Here's how the part is built. I have some questions about the finished solid (model axes, mm). A direction names the side the tool comes from. Give positions to 0.01 mm unless a question says otherwise; leave off trailing zeros. Write each loop counter-clockwise with the first axis right and the second up, starting at its lowest first coordinate (ties: lowest second). Pieces come first, ordered by that corner, then holes. Notation, with made-up numbers: (-21, 37.5) - (29, 37.5) arc R14 ccw to (29, 64.5) - close; hole circle Ø3 at (87.25, 23.5). An arc over 180 degrees is marked (long way). One line per item, written item: value. Start each with the question number.
1) On a 3-axis mill with a long thin cutter (end or side, diameter ignored), from which of +Z, -Z, +X, -X, +Y, -Y can I reach the whole of each face in a straight line? I mean faces 1 (the flat face through (-45.334, -78, -5)), 2 (the flat face through (-29, -84.507, 1)), 3 (the flat face through (-20, -78, 0.6)), 4 (the flat face through (-47.834, -78, -5)). Say none if no direction works.
2) Please list where these lines run through material, in increasing order: L1, parallel to X at y = -79.5, z = -0.5; L2, parallel to X at y = -72.5, z = 2.25; L3, parallel to Z at x = -19.5, y = -72.5. Write a range as [from, to].
3) I'm going to push flat-ended pins straight in: P1, Ø5, axis at y = -78.5, z = -6.5, coming from the -X side; P2, Ø9, axis at x = -37, y = -80.5, coming from the -Z side; P3, Ø1.2, axis at x = -28.5, y = -80.5, coming from the +Z side. Where does each tip first touch, or does it pass through?
4) Imagine slicing it at B-B on x = -29.5. Write out the boundary of the cut face in (y, z), plus the area to 3 significant figures.
5) Imagine slicing it at A-A on y = -73.5. Write out the boundary of the cut face in (x, z).
6) Imagine slicing it at C-C on z = 2.5. Write out the boundary of the cut face in (x, y).
from build123d import *

# Parameters (mm, degrees)
SKETCH_1_W      = 18
SKETCH_1_H      = 18.2
EXTRUDE_1_DEPTH = 3.4
SKETCH_2_W      = 2.5
SKETCH_2_H      = 15
EXTRUDE_2_DEPTH = 10
SKETCH_3_W      = 2.5
SKETCH_3_H      = 13.8
EXTRUDE_3_DEPTH = 1.8
SKETCH_4_W      = 15
SKETCH_4_H      = 11
EXTRUDE_4_DEPTH = 0.6


with BuildPart() as part:
    # 草圖1 → 填料-伸長1 (new body)
    with BuildSketch(Plane.XY):
        with Locations((-39.034480155, -77.607444045)):
            Rectangle(SKETCH_1_W, SKETCH_1_H)
    extrude(amount=EXTRUDE_1_DEPTH)

    # 草圖2 → 填料-伸長2 (add)
    with BuildSketch(Plane(origin=(0, 0, 0), x_dir=(-1, 0, 0), z_dir=(0, 0, -1))):
        with Locations((46.584480155, -77.607444045)):
            Rectangle(SKETCH_2_W, SKETCH_2_H)
    extrude(amount=EXTRUDE_2_DEPTH)

    # 草圖3 → 填料-伸長3 (add)
    with BuildSketch(Plane(origin=(0, 0, 0), x_dir=(-1, 0, 0), z_dir=(0, 0, -1))):
        with Locations((28.784480155, -77.607444045)):
            Rectangle(SKETCH_3_W, SKETCH_3_H)
    extrude(amount=-EXTRUDE_3_DEPTH)

    # 草圖4 → 填料-伸長4 (add)
    with BuildSketch(Plane(origin=(0, 0, 0), x_dir=(-1, 0, 0), z_dir=(0, 0, -1))):
        with Locations((20.034480155, -77.607444045)):
            Rectangle(SKETCH_4_W, SKETCH_4_H)
    extrude(amount=-EXTRUDE_4_DEPTH)


solid = part.part
Numbers:
1. face 1: -Z, +X, +Y, -Y
1. face 2: +Z, -Z, +X, -Y
1. face 3: +Z, +X, +Y, -Y
1. face 4: -Z, -X, +Y, -Y
2. L1: [-47.83, -45.33]
2. L2: [-48.03, -30.03]
2. L3: [0, 0.6]
3. P1: x = -47.83
3. P2: z = 0
3. P3: z = 1.8
4. outline: (-84.51, 0) - (-70.71, 0) - (-70.71, 1.8) - (-84.51, 1.8) - close
4. area: 24.8 mm^2
5. outline: (-48.03, 0) - (-47.83, 0) - (-47.83, -10) - (-45.33, -10) - (-45.33, 0) - (-12.53, 0) - (-12.53, 0.6) - (-27.53, 0.6) - (-27.53, 1.8) - (-30.03, 1.8) - (-30.03, 3.4) - (-48.03, 3.4) - close
6. outline: (-48.03, -86.71) - (-30.03, -86.71) - (-30.03, -68.51) - (-48.03, -68.51) - close
